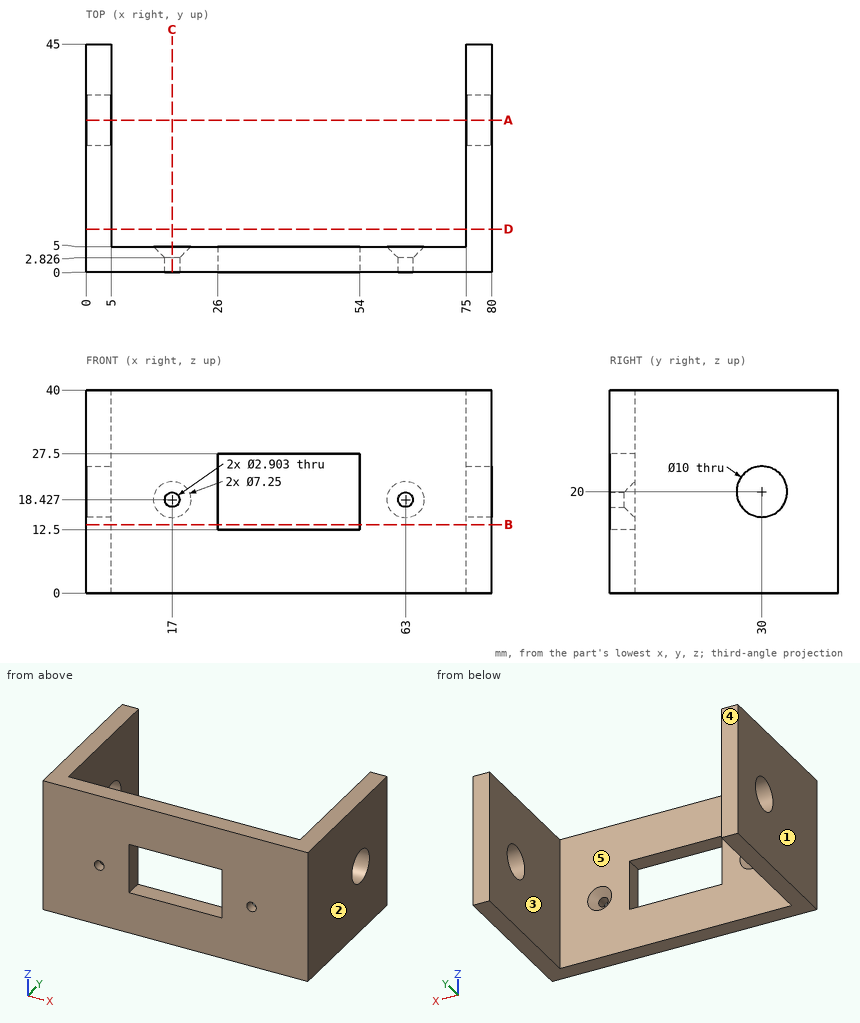
Verification items for this drawing (mm, ordinates from the low corner). A direction names the side the tool comes from. Give positions to 0.01 mm unless a question says otherwise; leave off trailing zeros. Loops run counter-clockwise (first coordinate to the right, second up) from the corner with the lowest first, then second, coordinate; pieces in that order, holes last. Notation, with made-up numbers: M 66,87.5 L 111,87.5 A19 cw 111,94.5 Z; hole C 2.25,26.5 d7. An arc over 180 degrees is marked long. Write item = value, one per line. Start each with the question number.
1. Section check D-D, the plane y = 8.5. Enter the section's corners in (x, z), plus the area to 3 significant figures.
2. Section check B-B, the plane z = 13.5. Enter the section's corners in (x, y), plus the area to 3 significant figures.
3. Thickness scan on probe 1 along X at (y, z) = (41, 9.5); probe 2 along Y at (x, z) = (3, 20); probe 3 along Z at (x, y) = (17, 2) (1 decimal). Record the ranges inside material, lowest first.
4. Draft check along X on the marked faces 1, 2 and 3. Enter one of: +X half, -X half, draft (parallel to the pull), parting line (faces both ways), or undercut.
5. Section check A-A, the plane y = 30. Enter the section's corners in (x, z).
6. Go/stop test with flat-tipped pins: P1, Ø2.5, axis at x = 63, z = 18.43, coming from the -Y side; P2, Ø3, axis at x = 59, z = 12.5, coming from the +Y side. Record where each tip stops, or that it passes through.
7. Tool access check on the marked faces 4 and 5. Record the directions out of +Z, -Z, +X, -X, +Y, -Y that give a thin tool (end or side, any length) a straight path to the whole face; none if there is none.
8. Section check C-C, the plane x = 17. Enter the section's corners in (y, z) (1 decimal).
Values follow:
q1.outline = M 0,0 L 5,0 L 5,40 L 0,40 Z; M 75,0 L 80,0 L 80,40 L 75,40 Z
q1.area = 400 mm^2
q2.outline = M 0,0 L 26,0 L 26,5 L 5,5 L 5,45 L 0,45 Z; M 54,0 L 80,0 L 80,45 L 75,45 L 75,5 L 54,5 Z
q2.area = 660 mm^2
q3.probe_1 = 0 to 5, 75 to 80
q3.probe_2 = 0 to 25, 35 to 45
q3.probe_3 = 0 to 17, 19.9 to 40
q4.face_1 = -X half
q4.face_2 = +X half
q4.face_3 = undercut
q5.outline = M 0,0 L 5,0 L 5,15 L 0,15 Z; M 0,25 L 5,25 L 5,40 L 0,40 Z; M 75,0 L 80,0 L 80,15 L 75,15 Z; M 75,25 L 80,25 L 80,40 L 75,40 Z
q6.P1 = through
q6.P2 = 5
q7.face_4 = +Z, -Z, +X, -X, +Y
q7.face_5 = +Z, -Z, +Y
q8.outline = M 0,0 L 5,0 L 5,14.8 L 2.8,17 L 0,17 Z; M 0,19.9 L 2.8,19.9 L 5,22.1 L 5,40 L 0,40 Z
